```python
from build123d import *

# Parameters (mm, degrees)
F2_R     = 7.5
F3_DEPTH = 33
F4_R     = 32
F5_DEPTH = 35.3


with BuildPart() as f1:
    # F0 (on Right) → F1 (revolve)
    with BuildSketch(Plane.YZ):
        with BuildLine():
            Line((0, 39), (0, 31))
            Line((0, 31), (30, 29))
            Line((30, 29), (30, 26))
            Line((30, 26), (72, 26))
            Line((72, 26), (72, 0))
            Line((72, 0), (90, 0))
            Line((90, 0), (90, 32))
            Line((90, 32), (93, 32))
            Line((93, 32), (93, 39))
            Line((93, 39), (60, 39))
            Line((60, 39), (45.8678821818, 29.1045845728))
            ThreePointArc((45.8678821818, 29.1045845728), (40.6912569338, 28.7652906284), (38, 33.2003447942))
            Line((38, 33.2003447942), (38, 45))
            Line((38, 45), (8, 45))
            Line((8, 45), (8, 39))
            Line((8, 39), (0, 39))
        make_face()
    revolve(axis=Axis((0, 81, 0), (0, -1, 0)))

    # F2 (on face) → F3 (join)
    with BuildSketch(Plane(origin=(0, 93, 0), x_dir=(-1, 0, 0), z_dir=(0, 1, 0))):
        with BuildLine():
            Line((36.2664732052, 14.3437415362), (19, 58))
            ThreePointArc((19, 58), (0, 77), (-19, 58))
            Line((-19, 58), (-36.2664732052, 14.3437415362))
            ThreePointArc((-36.2664732052, 14.3437415362), (0, 39), (36.2664732052, 14.3437415362))
        make_face()
        with BuildLine():
            ThreePointArc((0, 65.5), (5.3033008589, 63.3033008589), (7.5, 58))
            ThreePointArc((7.5, 58), (-5.3033008589, 52.6966991411), (0, 65.5))
        make_face(mode=Mode.SUBTRACT)
        with BuildLine():
            ThreePointArc((36.2188499541, -14.463571758), (0, -39), (-36.2188499541, -14.463571758))
            Line((-36.2188499541, -14.463571758), (-19, -57.5820319355))
            ThreePointArc((-19, -57.5820319355), (0, -76.5820319355), (19, -57.5820319355))
            Line((19, -57.5820319355), (36.2188499541, -14.463571758))
        make_face()
        with Locations((0, -57.5820319355)):
            Circle(F2_R, mode=Mode.SUBTRACT)
    extrude(amount=-F3_DEPTH)

    # F4 (on face) → F5 (cut)
    with BuildSketch(Plane(origin=(0, 90, 0), x_dir=(-1, 0, 0), z_dir=(0, 1, 0))):
        Circle(F4_R)
    extrude(amount=-F5_DEPTH, mode=Mode.SUBTRACT)


solid = f1.part
```
Check sheet for the modelled part. Datum: model origin and axes. Units: mm. A direction names the side the tool comes from. Round coordinates to 2 decimals unless told otherwise and drop trailing zeros. Write each loop counter-clockwise with the first axis right and the second up, starting at its lowest first coordinate (ties: lowest second). Pieces come first, ordered by that corner, then holes. Notation, with made-up numbers: (-14, -23.75) -> (3, -23.75) arc R23 cw to (3, 15.25) -> close; hole circle Ø11 at (73, 45). An arc over 180 degrees is marked (long way). One line per question, with ' | ' between items. Start each with the question number.
1. Set-up check for faces 1 (the face through (-27.5, 76.7, -36.3)), 2 (the face through (0.1, 54.7, 26.2)), 3 (the face through (27.51, 76.73, 36.48)), 4 (the face through (39, 76, 0)), 5 (the face through (-37, 8, -14)): record each of +Z, -Z, +X, -X, +Y, -Y from which the full face is reachable in a straight line by a thin tool's end or side.
2. Scan lines: line 1 along Z through (x, y) = (0, 69); line 2 along Y through (x, z) = (-14.5, 42); line 3 along Z through (x, y) = (-1, 31.5). Record each from-to range of solid material in increasing order. Write a range as from..to.
3. Sectioned sample at A-A, the plane z = 43. Record the cut outline in (x, y).
4. Release check for a two-part mould opening along X. For faces 6 (the face through (-39, 76, 0)), 7 (the face through (-1.301, 46.554, -29.556)), 8 (the face through (15.821, 42.523, -20.633)) record: +X half, -X half, draft (parallel to the pull), parting line (faces both ways), or undercut.
5. Sectioned sample at B-B, the plane y = 69. Record the cut outline in (x, z), then the cut area to 3 significant figures.
6. Sectioned sample at D-D, the plane z = 60. Record the cut outline in (x, y).
7. Sectioned sample at C-C, the plane y = 16.5. Record the cut outline in (x, z).
8. Depth check by flat-ended pin: pin 1 (6 mm diameter, centred on y = 36, z = 34.5, fed in from +X); pin 2 (18.5 mm diameter, centred on x = -2, z = -60.5, fed in from -Y); pin 3 (1.5 mm diameter, centred on x = 35, z = -3.5, fed in from -Y); pin 4 (1.5 mm diameter, centred on x = 22.5, y = 35, fed in from +Z). Enter the tip coordinate at first touch or a pass-through.
Taken from the geometry:
1) face 1: -Z, -X, +Y | face 2: +Y | face 3: +Z, +X, +Y | face 4: +X, +Y | face 5: -Y
2) line 1: z = -76.58..-65.08, -50.08..-32, 32..50.5, 65.5..77 | line 2: y = 8..38, 60..93 | line 3: z = -44.99..-25.98, 25.98..44.99
3) outline: (-24.93, 60) -> (24.93, 60) -> (24.93, 93) -> (-24.93, 93) -> close; (-13.27, 8) -> (13.27, 8) -> (13.27, 38) -> (-13.27, 38) -> close
4) face 6: -X half | face 7: parting line | face 8: undercut
5) outline: (-36.27, 14.34) arc R39 ccw to (-36.22, -14.46) -> (-19, -57.58) arc R19 ccw to (19, -57.58) -> (36.22, -14.46) arc R39 ccw to (36.27, 14.34) -> (19, 58) arc R19 ccw to (-19, 58) -> close; hole circle Ø64 at (0, 0); hole circle Ø15 at (0, -57.58); hole circle Ø15 at (0, 58) | area: 4,550 mm^2
6) outline: (-18.89, 60) -> (-7.23, 60) -> (-7.23, 93) -> (-18.89, 93) -> close; (7.23, 60) -> (18.89, 60) -> (18.89, 93) -> (7.23, 93) -> close
7) outline: circle Ø90 at (0, 0); hole circle Ø59.8 at (0, 0)
8) pin 1: stops at x = 32.14 | pin 2: stops at y = 60 | pin 3: stops at y = 0 | pin 4: stops at z = 39.39
